from build123d import *

# Parameters (mm, degrees)
F0_R     = 9
F1_DEPTH = 50
F2_R     = 9
F2_R_2   = 6.5
F3_DEPTH = 3
F5_D     = 6.8
F5_DEPTH = 20
F5_TIP   = 2.0429261047
F7_D     = 12
F7_DEPTH = 30
F7_TIP   = 3.6051637142


with BuildPart() as f1:
    # F0 (on Front) → F1 (new body)
    with BuildSketch(Plane.XZ):
        Circle(F0_R)
    extrude(amount=F1_DEPTH)

    # F2 (on face) → F3 (cut)
    with BuildSketch(Plane.XZ.offset(50)):
        Circle(F2_R)
        Circle(F2_R_2, mode=Mode.SUBTRACT)
    extrude(amount=-F3_DEPTH, mode=Mode.SUBTRACT)

    # F5
    with Locations(Plane.XZ.offset(50)):
        with Locations((0, 0)):
            Hole(F5_D / 2, depth=F5_DEPTH)
            with Locations((0, 0, -(F5_DEPTH + F5_TIP / 2))):  # 118° drill point
                Cone(0, F5_D / 2, F5_TIP, mode=Mode.SUBTRACT)

    # F7
    with Locations(Plane(origin=(0, 0, 0), x_dir=(-1, 0, 0), z_dir=(0, 1, 0))):
        with Locations((0, 0)):
            Hole(F7_D / 2, depth=F7_DEPTH)
            with Locations((0, 0, -(F7_DEPTH + F7_TIP / 2))):  # 118° drill point
                Cone(0, F7_D / 2, F7_TIP, mode=Mode.SUBTRACT)


solid = f1.part
Geometry check sheet. Reference: the model listing, model coordinates, mm. A direction names the side the tool comes from. Round coordinates to 2 decimals unless told otherwise and drop trailing zeros. Order: outer loops, then holes, each group sorted by start corner. A loop starts at its lowest first (then second) coordinate and runs counter-clockwise, first axis right, second up. Notation, with made-up numbers: M -3.5,35.25 L 52.5,35.25 A17 cw 52.5,66.25 Z; hole C 47,-11.75 d11. An arc over 180 degrees is marked long. Answer in a Markdown table with one row per item. Add a question column.
Item 1: Sectioned sample at C-C, the plane y = -28. Enter the section's corners in (x, z), plus the area to 3 significant figures.
Item 2: Set-up check for faces 4 (the face through (3, -47, -6)), 5 (the face through (-6, -15, 0)), 6 (the face through (-1.172, -23.171, 8.923)): record each of +Z, -Z, +X, -X, +Y, -Y from which the full face is reachable in a straight line by a thin tool's end or side.
Item 3: Sectioned sample at D-D, the plane x = -7.5. Enter the section's corners in (y, z).
Item 4: Material ranges on L1, parallel to Z at x = 0, y = -41; L2, parallel to Z at x = 0, y = -13.75; L3, parallel to Y at x = -4.5, z = 5.5, recorded low to high. Write a range as [from, to].
Item 5: Sectioned sample at A-A, the plane x = 0. Enter the section's corners in (y, z).
Item 6: Depth check by flat-ended pin: pin 1 Ø3 at (x, z) = (5.5, 6.5) entering from -Y; pin 2 Ø1.5 at (x, z) = (5, -0.5) entering from +Y; pin 3 Ø2 at (x, y) = (-2, -36.5) entering from -Z. Enter the tip coordinate at first touch or a pass-through.
Item 7: Draft check along Z on faces 1 (the face through (-5.158, -48.521, -3.955)), 2 (the face through (3, -50, -3)), 3 (the face through (0.74, -40.65, -3.32)). Enter one of: released by +Z, released by -Z, zero draft, split by the parting line, or undercut.
Item 8: Sectioned sample at B-B, the plane z = 0. Enter the section's corners in (x, y), plus the area to 3 significant figures.
Filled in:
| question | item | result |
|---|---|---|
| 1 | outline | C 0,0 d18; hole C 0,0 d12 |
| 1 | area | 141 mm² |
| 2 | face 4 | -Y |
| 2 | face 5 | +Y |
| 2 | face 6 | +Y, -Y |
| 3 | outline | M -47,-4.97 L 0,-4.97 L 0,4.97 L -47,4.97 Z |
| 4 | L1 | z = [-9, -3.4], [3.4, 9] |
| 4 | L2 | z = [-9, -6], [6, 9] |
| 4 | L3 | y = [-47, 0] |
| 5 | outline | M -50,-6.5 L -47,-6.5 L -47,-9 L 0,-9 L 0,-6 L -30,-6 L -31.56,-3.4 L -50,-3.4 Z; M -50,3.4 L -31.56,3.4 L -30,6 L 0,6 L 0,9 L -47,9 L -47,6.5 L -50,6.5 Z |
| 6 | pin 1 | stops at y = -47 |
| 6 | pin 2 | stops at y = -30.14 |
| 6 | pin 3 | stops at z = -8.94 |
| 7 | face 1 | split by the parting line |
| 7 | face 2 | zero draft |
| 7 | face 3 | undercut |
| 8 | outline | M -9,-47 L -6.5,-47 L -6.5,-50 L -3.4,-50 L -3.4,-31.56 L -6,-30 L -6,0 L -9,0 Z; M 3.4,-50 L 6.5,-50 L 6.5,-47 L 9,-47 L 9,0 L 6,0 L 6,-30 L 3.4,-31.56 Z |
| 8 | area | 385 mm² |
